from build123d import *

# Parameters (mm, degrees)
SCHIZZO1_R                   = 1.75
SCHIZZO1_R_2                 = 11.05
ESTRUSIONE_ESTRUSIONE1_DEPTH = 2
SCHIZZO14_W                  = 20
SCHIZZO14_H                  = 2
ESTRUSIONE_ESTRUSIONE2_DEPTH = 22
SCHIZZO15_R                  = 2.5
TAGLIO_ESTRUSIONE1_DEPTH     = 10
SMUSSO1_SIZE                 = 10
RACCORDO1_R                  = 2
CONVERTI_SOLIDO2_START       = -49.5
CONVERTI_SOLIDO2_OUTLINE_R   = 2.5
CONVERTI_SOLIDO2_DEPTH       = 4
BORDO_FLANGIA1_START         = -10
BORDO_FLANGIA1_DEPTH         = 20
SCHIZZO27_R                  = 2.5
TAGLIO_ESTRUSIONE2_DEPTH     = 10
RACCORDO3_R                  = 2


# Read off the part's stored shape, not the designer's step: Converti-Solido2, Bordo-Flangia1
with BuildPart() as part:
    # Schizzo1 → Estrusione-Estrusione1 (new body)
    with BuildSketch(Plane.XY):
        Polygon((-25, -27.5), (-10, -27.5), (-10, -49.5), (10, -49.5), (10, -27.5), (25, -27.5), (25, 27.5), (-25, 27.5), align=None)
        with Locations((-15.5, 15.5)):
            Circle(SCHIZZO1_R, mode=Mode.SUBTRACT)
        with Locations((15.5, 15.5)):
            Circle(SCHIZZO1_R, mode=Mode.SUBTRACT)
        with Locations((15.5, -15.5)):
            Circle(SCHIZZO1_R, mode=Mode.SUBTRACT)
        with Locations((-15.5, -15.5)):
            Circle(SCHIZZO1_R, mode=Mode.SUBTRACT)
        Circle(SCHIZZO1_R_2, mode=Mode.SUBTRACT)
    extrude(amount=ESTRUSIONE_ESTRUSIONE1_DEPTH)

    # Schizzo14 → Estrusione-Estrusione2 (add)
    with BuildSketch(Plane.XY.offset(2)):
        with Locations((0, -48.5)):
            Rectangle(SCHIZZO14_W, SCHIZZO14_H)
    extrude(amount=ESTRUSIONE_ESTRUSIONE2_DEPTH)

    # Schizzo15 → Taglio-Estrusione1 (cut)
    with BuildSketch(Plane(origin=(0, -47.5, 0), x_dir=(1, 0, 0), z_dir=(0, 1, 0))):
        with Locations(Location((0, -14, 0), (0, 0, 270))):
            Circle(SCHIZZO15_R)
    extrude(amount=-TAGLIO_ESTRUSIONE1_DEPTH, mode=Mode.SUBTRACT)

    # Smusso1
    smusso1_edges = [part.edges().sort_by_distance(p)[0] for p in [
        (25, -27.5, 1),
        (-25, -27.5, 1),
        (-25, 27.5, 1),
        (25, 27.5, 1),
    ]]
    chamfer(smusso1_edges, length=SMUSSO1_SIZE)

    # Raccordo1
    raccordo1_edges = [part.edges().sort_by_distance(p)[0] for p in [
        (10, -27.5, 1),
        (-10, -27.5, 1),
        (0, -47.5, 2),
        (-10, -48.5, 24),
        (10, -48.5, 24),
        (0, -49.5, 0),
    ]]
    fillet(raccordo1_edges, radius=RACCORDO1_R)

    # Converti-Solido2 outline → Converti-Solido2 (cut)
    with BuildSketch(Plane(origin=(0, 0, 0), x_dir=(1, 0, 0), z_dir=(0, 1, 0)).offset(CONVERTI_SOLIDO2_START)):
        with BuildLine():
            Line((-10, 0), (-10, -22))
            ThreePointArc((-10, -22), (-9.414213562, -23.414213562), (-8, -24))
            Line((-8, -24), (8, -24))
            ThreePointArc((8, -24), (9.414213562, -23.414213562), (10, -22))
            Line((10, -22), (10, 0))
            Line((10, 0), (-10, 0))
        make_face()
        with Locations((0, -14)):
            Circle(CONVERTI_SOLIDO2_OUTLINE_R, mode=Mode.SUBTRACT)
    extrude(amount=CONVERTI_SOLIDO2_DEPTH, mode=Mode.SUBTRACT)

    # Bordo-Flangia1 outline → Bordo-Flangia1 (add)
    with BuildSketch(Plane.YZ.offset(BORDO_FLANGIA1_START)):
        with BuildLine():
            ThreePointArc((-47.5, 2), (-46.914213562, 0.585786438), (-45.5, 0))
            Line((-45.5, 0), (-45.5, 22))
            Line((-45.5, 22), (-47.5, 22))
            Line((-47.5, 22), (-47.5, 2))
        make_face()
    extrude(amount=BORDO_FLANGIA1_DEPTH)

    # Schizzo27 → Taglio-Estrusione2 (cut)
    with BuildSketch(Plane(origin=(0, -45.5, 0), x_dir=(1, 0, 0), z_dir=(0, 1, 0))):
        with Locations(Location((0, -14, 0), (0, 0, 270))):
            Circle(SCHIZZO27_R)
    extrude(amount=-TAGLIO_ESTRUSIONE2_DEPTH, mode=Mode.SUBTRACT)

    # Raccordo3
    raccordo3_edges = [part.edges().sort_by_distance(p)[0] for p in [
        (10, -46.5, 22),
        (-10, -46.5, 22),
    ]]
    fillet(raccordo3_edges, radius=RACCORDO3_R)


solid = part.part
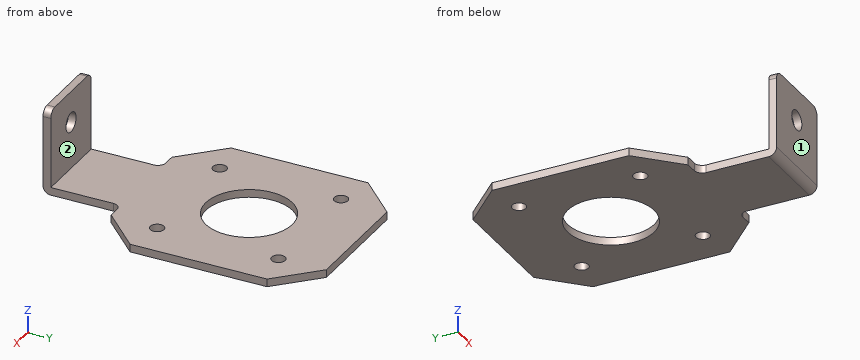
The model under review builds one solid part; all positions refer to its coordinate system, in mm. Face numbers are marked on the shaded views. A direction names the side the tool comes from. Give positions to 0.01 mm unless a question says otherwise; leave off trailing zeros. Order: outer loops, then holes, each group sorted by start corner. A loop starts at its lowest first (then second) coordinate and runs counter-clockwise, first axis right, second up. Notation, with made-up numbers: M -32,47.5 L 6,47.5 A24 cw 6,78.5 Z; hole C 34,49.25 d3. An arc over 180 degrees is marked long. Use one line per item in the form item = value. Start each with the question number.
Item 1: We need section B-B on z = 14. Give the boundary of the cut face in (x, y).
Item 2: For the marked faces 1 and 2, list the 3-axis set-ups (+Z, -Z, +X, -X, +Y, -Y) from which the entire face can be reached by the end or side of a thin tool; tool diameter is ignored.
Item 3: Insertion check: pin 1 Ø1.6 at (x, z) = (-14, 1) entering from -Y; pin 2 Ø3 at (x, y) = (15.5, -15.5) entering from -Z; pin 3 Ø12 at (x, z) = (10, 9) entering from +Y. Each pin has a flat end and moves straight along its axis. Give the tip position at first contact, or say it passes through.
Item 4: We need section A-A on y = 15.5. Give the boundary of the cut face in (x, z), plus the area to 3 significant figures.
Item 5: We need section D-D on x = 6. Give the boundary of the cut face in (y, z).
Item 6: We need section C-C on y = 0. Give the boundary of the cut face in (x, z), plus the area to 3 significant figures.
Item 7: To check wall thickness, follow line 1 along Y through (x, z) = (-15.5, 1); line 2 along Z through (x, y) = (11.5, 4.5); line 3 along Y through (x, z) = (0, 7.5). State the ranges of each line that lie inside material, in increasing order. Write a range as from..to.
Completed:
q1.outline = M -10,-47.5 L -2.5,-47.5 L -2.5,-45.5 L -10,-45.5 Z; M 2.5,-47.5 L 10,-47.5 L 10,-45.5 L 2.5,-45.5 Z
q2.face_1 = +Z, -Z, +X, -X, -Y
q2.face_2 = +Z, +X, -X, +Y
q3.pin_1 = -27.5
q3.pin_2 = through
q3.pin_3 = -45.5
q4.outline = M -25,0 L -17.25,0 L -17.25,2 L -25,2 Z; M -13.75,0 L 13.75,0 L 13.75,2 L -13.75,2 Z; M 17.25,0 L 25,0 L 25,2 L 17.25,2 Z
q4.area = 86.0 mm²
q5.outline = M -47.5,2 A2 ccw -45.5,0 L -9.28,0 L -9.28,2 L -45.5,2 L -45.5,22 L -47.5,22 Z; M 9.28,0 L 27.5,0 L 27.5,2 L 9.28,2 Z
q6.outline = M -25,0 L -11.05,0 L -11.05,2 L -25,2 Z; M 11.05,0 L 25,0 L 25,2 L 11.05,2 Z
q6.area = 55.8 mm²
q7.line_1 = -27..-17.25, -13.75..13.75, 17.25..27
q7.line_2 = 0..2
q7.line_3 = -47.5..-45.5
